Design review of the part built by this model. Coordinates are the model's own, in mm. A direction names the side the tool comes from. Give positions to 0.01 mm unless a question says otherwise; leave off trailing zeros. Write each loop counter-clockwise with the first axis right and the second up, starting at its lowest first coordinate (ties: lowest second). Pieces come first, ordered by that corner, then holes. Notation, with made-up numbers: (22, 35) -> (74, 35) arc R10 cw to (74, 45) -> close; hole circle Ø9 at (39, 36). An arc over 180 degrees is marked (long way). Answer as a JSON object with one key per item and string values.
```python
from build123d import *

# Parameters (mm, degrees)
SKETCH1_R           = 46
SKETCH1_R_2         = 40
BOSS_EXTRUDE1_DEPTH = 961
SKETCH2_W           = 170
SKETCH2_H           = 170
SKETCH2_R           = 9
BOSS_EXTRUDE2_DEPTH = 12
SKETCH3_W           = 170
SKETCH3_H           = 170
SKETCH3_R           = 9
BOSS_EXTRUDE3_DEPTH = 12


with BuildPart() as part:
    # Sketch1 → Boss-Extrude1 (new body)
    with BuildSketch(Plane.XY):
        Circle(SKETCH1_R)
        Circle(SKETCH1_R_2, mode=Mode.SUBTRACT)
    extrude(amount=BOSS_EXTRUDE1_DEPTH)

    # Sketch2 → Boss-Extrude2 (add)
    with BuildSketch(Plane(origin=(0, 0, 0), x_dir=(-1, 0, 0), z_dir=(0, 0, -1))):
        Rectangle(SKETCH2_W, SKETCH2_H)
        with Locations((64.227589169, 0)):
            Circle(SKETCH2_R, mode=Mode.SUBTRACT)
        with Locations((-68.030538528, 0)):
            Circle(SKETCH2_R, mode=Mode.SUBTRACT)
        with Locations((60.407969797, 46.896616819)):
            Circle(SKETCH2_R, mode=Mode.SUBTRACT)
        with Locations((25.416815813, 60.663628222)):
            Circle(SKETCH2_R, mode=Mode.SUBTRACT)
    extrude(amount=BOSS_EXTRUDE2_DEPTH)

    # Sketch3 → Boss-Extrude3 (add)
    with BuildSketch(Plane.XY.offset(961)):
        Rectangle(SKETCH3_W, SKETCH3_H)
        with Locations((47.306709653, 56.060313407)):
            Circle(SKETCH3_R, mode=Mode.SUBTRACT)
        with Locations((-23.467107938, 60.902732505)):
            Circle(SKETCH3_R, mode=Mode.SUBTRACT)
        with Locations((-60.716485617, 46.226195512)):
            Circle(SKETCH3_R, mode=Mode.SUBTRACT)
        with Locations((-64.441423385, -32.965699246)):
            Circle(SKETCH3_R, mode=Mode.SUBTRACT)
    extrude(amount=BOSS_EXTRUDE3_DEPTH)


solid = part.part
```
(1) We need section B-B, the plane x = 0. State the section outline as (y, z) points.
Here are the results:
{"outline": "(-85, -12) -> (85, -12) -> (85, 0) -> (46, 0) -> (46, 961) -> (85, 961) -> (85, 973) -> (-85, 973) -> (-85, 961) -> (-46, 961) -> (-46, 0) -> (-85, 0) -> close; hole (-40, 0) -> (40, 0) -> (40, 961) -> (-40, 961) -> close"}
(2) Clearance check with flat-ended pins moving along their axes: pin 1 (11 mm diameter, centred on x = -25.42, y = 60.66, fed in from -Z); pin 2 (5 mm diameter, centred on y = 7.5, z = 188.5, fed in from -X); pin 3 (4 mm diameter, centred on x = 37.5, z = 677.5, fed in from -Y); pin 4 (1.5 mm diameter, centred on y = 20, z = 259, fed in from -X). State where each tip first meets the part, or that it passes through.
Here are the results:
{"pin 1": "passes through", "pin 2": "stops at x = -45.73", "pin 3": "stops at y = -29.25", "pin 4": "stops at x = -41.78"}
(3) For faces 1 (the flat face through (39, -37, 0)), 2 (the flat face through (-1, 1, 973)), 3 (the cylindrical face through (-72.812, 2.703, -5.916)), 4 (the cylindrical face through (51.46, 48.076, 966.916)), list the 3-axis set-ups (+Z, -Z, +X, -X, +Y, -Y) from which the entire face can be reached by the end or side of a thin tool; tool diameter is ignored.
Here are the results:
{"face 1": "none", "face 2": "+Z, +X, -X, +Y, -Y", "face 3": "-Z", "face 4": "+Z"}
(4) We need section A-A, the plane y = 0. State the section outline as (x, z) points, then the cut area to 3 significant figures.
Here are the results:
{"outline": "(-85, -12) -> (-73.23, -12) -> (-73.23, 0) -> (-85, 0) -> close; (-85, 961) -> (-46, 961) -> (-46, 0) -> (-55.23, 0) -> (-55.23, -12) -> (59.03, -12) -> (59.03, 0) -> (46, 0) -> (46, 961) -> (85, 961) -> (85, 973) -> (-85, 973) -> close; (77.03, -12) -> (85, -12) -> (85, 0) -> (77.03, 0) -> close; hole (-40, 0) -> (40, 0) -> (40, 961) -> (-40, 961) -> close", "area": "15,200 mm²"}
(5) We need section C-C, the plane z = 458. State the section outline as (x, y) points, then the cut area to 3 significant figures.
Here are the results:
{"outline": "circle Ø92 at (0, 0); hole circle Ø80 at (0, 0)", "area": "1,620 mm²"}
(6) For line 1 along Z through (x, y) = (-33.5, 10.5); line 2 along Y through (x, z) = (1.5, 457); line 3 along Y through (x, z) = (-12.5, 606), list the stretches that pass through material, from the lowest coordinate up.
Here are the results:
{"line 1": "z = -12 to 0, 961 to 973", "line 2": "y = -45.98 to -39.97, 39.97 to 45.98", "line 3": "y = -44.27 to -38, 38 to 44.27"}
(7) The part is to be moulded in two halves that separate along Z. For faces 5 (the cylindrical face through (77.02, 0.4, -5.92)), 6 (the flat face through (1, 1, -12)), 7 (the flat face through (1, 1, 0)), say which applies: +Z half, -Z half, draft (parallel to the pull), parting line (faces both ways), or undercut.
Here are the results:
{"face 5": "draft", "face 6": "-Z half", "face 7": "undercut"}
